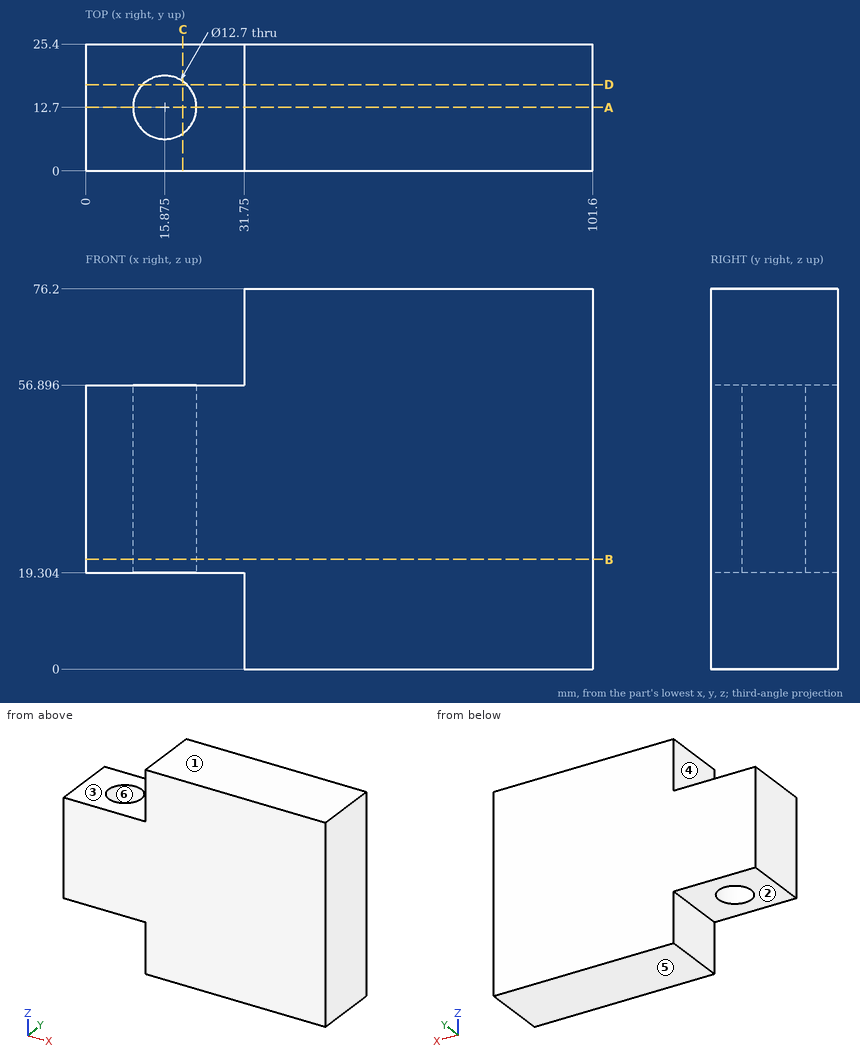
Geometry: see drawing. Coordinates: mm, zero at the bounding-box minimum. A direction names the side the tool comes from. Coordinates: 2 decimals unless noted, no trailing zeros. Write each loop counter-clockwise with the first axis right and the second up, starting at its lowest first coordinate (ties: lowest second). Pieces come first, ordered by that corner, then holes.
1) Material intervals for line 1 along Y through (x, z) = (16, 24.5); line 2 along Z through (x, y) = (23, 24.25); line 3 along X through (y, z) = (15.5, 73), sorted ascending.
2) Mould query, pull axis X, two halves, no side actions, for the marked faces 4, 5 and 6. Classes: pulls with the +X half, pulls with the -X half, needs draft (parallel to the pull), parting line crosses it, or undercut.
3) Section C-C on x = 19.5. Output: boundary loops of the cut face in (y, z).
4) Section B-B on z = 22. Output: boundary loops of the cut face in (x, y) (3 decimals).
5) Set-up query: the marked faces 1, 2 and 3. Return all of +Z, -Z, +X, -X, +Y, -Y with unobstructed straight access to the full face (end or side cutting, diameter ignored); none if empty.
6) Section A-A on y = 12.7. Output: boundary loops of the cut face in (x, z) (3 decimals), and give its area (3 significant figures).
7) Section D-D on y = 17.25. Output: boundary loops of the cut face in (x, z).
8) Pin query (flat end, axial travel): pin 1 Ø7.5 at (x, y) = (18.5, 8.5) entering from -Z; pin 2 Ø6 at (y, z) = (15, 65) entering from -X; pin 3 Ø12 at (x, y) = (32.5, 12) entering from -Z. Return the tip coordinate at first contact, or that it passes through.
Check result:
1. line 1: y = 0 to 6.35, 19.05 to 25.4
1. line 2: z = 19.3 to 56.9
1. line 3: x = 31.75 to 101.6
2. face 4: pulls with the -X half
2. face 5: needs draft
2. face 6: undercut
3. outline: (0, 19.3) - (7.49, 19.3) - (7.49, 56.9) - (0, 56.9) - close; (17.91, 19.3) - (25.4, 19.3) - (25.4, 56.9) - (17.91, 56.9) - close
4. outline: (0, 0) - (101.6, 0) - (101.6, 25.4) - (0, 25.4) - close; hole circle Ø12.7 at (15.875, 12.7)
5. face 1: +Z, +X, -X, +Y, -Y
5. face 2: -Z, -X, +Y, -Y
5. face 3: +Z, -X, +Y, -Y
6. outline: (0, 19.304) - (9.525, 19.304) - (9.525, 56.896) - (0, 56.896) - close; (22.225, 19.304) - (31.75, 19.304) - (31.75, 0) - (101.6, 0) - (101.6, 76.2) - (31.75, 76.2) - (31.75, 56.896) - (22.225, 56.896) - close
6. area: 6,040 mm2
7. outline: (0, 19.3) - (11.45, 19.3) - (11.45, 56.9) - (0, 56.9) - close; (20.3, 19.3) - (31.75, 19.3) - (31.75, 0) - (101.6, 0) - (101.6, 76.2) - (31.75, 76.2) - (31.75, 56.9) - (20.3, 56.9) - close
8. pin 1: stops at z = 19.3
8. pin 2: stops at x = 31.75
8. pin 3: stops at z = 0
